Source: CAD feature listing. Evaluate the final solid. Frame: model axes, mm. A direction names the side the tool comes from. Coordinates: 2 decimals unless noted, no trailing zeros. Write each loop counter-clockwise with the first axis right and the second up, starting at its lowest first coordinate (ties: lowest second). Pieces come first, ordered by that corner, then holes. Notation, with made-up numbers: (-10.75, 7.5) -> (47.25, 7.5) arc R17 cw to (47.25, 33.5) -> close; hole circle Ø5 at (48.25, 26). An arc over 180 degrees is marked (long way). One line per item, written item: value. Start each with the question number.
1. Section query C-C, the plane y = 63. Output: boundary loops of the cut face in (x, z) (1 decimal).
2. Section query B-B, the plane z = 2.25. Output: boundary loops of the cut face in (x, y) (1 decimal), and give its area (3 significant figures).
3. Section query D-D, the plane x = -0.75. Output: boundary loops of the cut face in (y, z).
4. First-contact query: P1, Ø4, axis at x = -5, y = 50.5, coming from the +Z side; P2, Ø1.9, axis at x = -4.76, y = 4.76, coming from the -Z side. Flat tips, straight axial feed; report the tip coordinate or a pass-through.
5. Mould query, pull axis Y, two halves, no side actions, for faces 1 (the flat face through (-8.72, 0.78, 0.78)), 2 (the flat face through (-5, 39, 1.588)), 3 (the flat face through (-5, 39, 0)). Classes: released by +Y, released by -Y, zero draft, split by the parting line, or undercut.
6. Line query: line 1 (Y direction, x = -5.5, z = 2.6); line 2 (X direction, y = 73, z = 1.75); line 3 (Z direction, x = -1.5, y = 65.5). Output: solid intervals per line, ascending.
7. Access query for faces 4 (the cylindrical face through (-5.28, 2.44, 3.15)), 5 (the flat face through (-5, 6, 4.762)). Directions: +Z, -Z, +X, -X, +Y, -Y. A direction counts if a zero-diameter tool reaches every point of the face in a straight line with its end or side. Return the directions, or none.
8. Section query A-A, the plane x = -5. Output: boundary loops of the cut face in (y, z).
from build123d import *
from build123d.topology import SkipClean

# Parameters (mm, degrees)
SKETCH1_W                    = 9.525
SKETCH1_H                    = 77.7875
BOSS_EXTRUDE1_DEPTH          = 1.5875
CHAMFER2_SIZE                = 1.5875
F_97_0_0825_DIAMETER_HOLE1_D = 2.0955
SKETCH5_R                    = 2.38125
SKETCH5_R_2                  = 1.04775
BOSS_EXTRUDE2_DEPTH          = 3.175


with BuildPart() as part:
    # Sketch1 → Boss-Extrude1 (new body)
    with BuildSketch(Plane.XY):
        with Locations((-4.7625, 38.89375)):
            Rectangle(SKETCH1_W, SKETCH1_H)
    extrude(amount=BOSS_EXTRUDE1_DEPTH)

    # Chamfer2
    chamfer2_edges = [part.edges().sort_by_distance(p)[0] for p in [
        (0, 0, 0.79375),
        (-9.525, 0, 0.79375),
        (-9.525, 77.7875, 0.79375),
        (0, 77.7875, 0.79375),
    ]]
    chamfer(chamfer2_edges, length=CHAMFER2_SIZE)

    # 97 _0.0825_ Diameter Hole1 (through all)
    with Locations(Plane.XY.offset(1.5875)):
        with Locations((-4.7625, 4.7625), (-4.7625, 73.025)):
            Hole(F_97_0_0825_DIAMETER_HOLE1_D / 2)

    # Sketch5 → Boss-Extrude2 (add)
    # profile 1 of 2: a face of its own
    with SkipClean():  # the faces are left unmerged after this step: merging them gives an invalid solid
        with BuildSketch(Plane.XY.offset(1.5875)):
            with Locations((-4.7625, 4.7625)):
                Circle(SKETCH5_R)
            with Locations((-4.7625, 4.7625)):
                Circle(SKETCH5_R_2, mode=Mode.SUBTRACT)
        # profile 2 of 2: a face of its own
        with BuildSketch(Plane.XY.offset(1.5875)):
            with Locations(Location((-4.7625, 73.025, 0), (0, 0, 180))):
                Circle(SKETCH5_R)
            with Locations((-4.7625, 73.025)):
                Circle(SKETCH5_R_2, mode=Mode.SUBTRACT)
        extrude(amount=BOSS_EXTRUDE2_DEPTH)
    add(part.part.scale(1), mode=Mode.REPLACE)  # the faces are merged on a copy


solid = part.part
Computed values:
1. outline: (-9.5, 0) -> (0, 0) -> (0, 1.6) -> (-9.5, 1.6) -> close
2. outline: circle Ø4.8 at (-4.8, 4.8); circle Ø4.8 at (-4.8, 73); hole circle Ø2.1 at (-4.8, 4.8); hole circle Ø2.1 at (-4.8, 73)
2. area: 28.7 mm²
3. outline: (0.84, 0) -> (76.95, 0) -> (76.95, 1.59) -> (0.84, 1.59) -> close
4. P1: stops at z = 1.59
4. P2: passes through
5. face 1: released by -Y
5. face 2: undercut
5. face 3: zero draft
6. line 1: y = 2.5 to 4.02, 5.51 to 7.03, 70.76 to 72.28, 73.77 to 75.29
6. line 2: x = -7.14 to -5.81, -3.72 to -2.38
6. line 3: z = 0 to 1.59
7. face 4: +Z
7. face 5: +Z, +X, -X, +Y, -Y
8. outline: (0, 0) -> (3.74, 0) -> (3.74, 4.76) -> (2.39, 4.76) -> (2.39, 1.59) -> (0, 1.59) -> close; (5.78, 0) -> (72, 0) -> (72, 4.76) -> (70.66, 4.76) -> (70.66, 1.59) -> (7.13, 1.59) -> (7.13, 4.76) -> (5.78, 4.76) -> close; (74.05, 0) -> (77.79, 0) -> (77.79, 1.59) -> (75.39, 1.59) -> (75.39, 4.76) -> (74.05, 4.76) -> close
